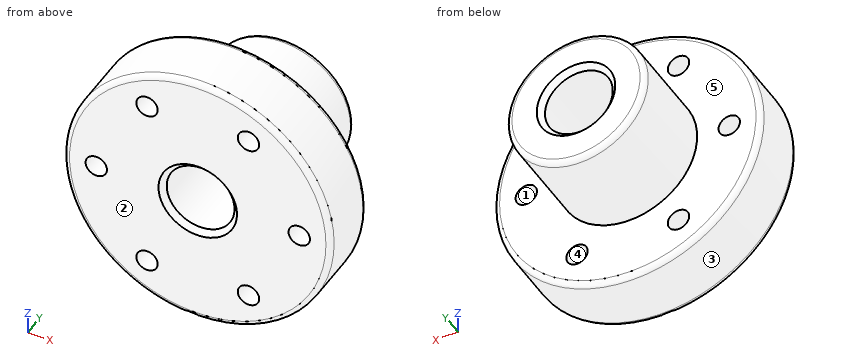
```python
from build123d import *

# Parameters (mm, degrees)
ESQUISSE3_R                  = 1
ENL_V_MAT_EXTRU_1_DEPTH      = 7
R_P_TITION_CIRCULAIRE1_COUNT = 6
CONG_1_R                     = 0.5
CHANFREIN1_SIZE              = 0.5


with BuildPart() as part:
    # Esquisse1 → Révolution2 (revolve)
    with BuildSketch(Plane.XY):
        Polygon((6.5, 15), (6.5, 6), (12.5, 6), (12.5, 0), (3.175, 0), (3.175, 15), align=None)
    revolve(axis=Axis((0, 0, 0), (0, 1, 0)))

    # Esquisse3 → Enlèv. mat.-Extru.1 (cut, through all)
    with BuildSketch(Plane(origin=(0, 6, 0), x_dir=(1, 0, 0), z_dir=(0, 1, 0))):
        with Locations((9.5, 0)):
            Circle(ESQUISSE3_R)
    enl_v_mat_extru_1 = extrude(amount=-ENL_V_MAT_EXTRU_1_DEPTH, mode=Mode.SUBTRACT)

    # Répétition circulaire1: Enlèv. mat.-Extru.1 ×6 about axis
    r_p_tition_circulaire1_axis = Axis((0, 0, 0), (0, 1, 0))
    for i in range(1, R_P_TITION_CIRCULAIRE1_COUNT):
        add(enl_v_mat_extru_1.rotate(r_p_tition_circulaire1_axis, i * 360 / R_P_TITION_CIRCULAIRE1_COUNT), mode=Mode.SUBTRACT)

    # Congé1
    cong_1_edges = [part.edges().sort_by_distance(p)[0] for p in [
        (-6.5, 15, 0),
        (-12.5, 6, 0),
        (-12.5, 0, 0),
    ]]
    fillet(cong_1_edges, radius=CONG_1_R)

    # Chanfrein1
    chanfrein1_edges = [part.edges().sort_by_distance(p)[0] for p in [
        (-3.175, 0, 0),
        (-3.175, 15, 0),
    ]]
    chamfer(chanfrein1_edges, length=CHANFREIN1_SIZE)


solid = part.part
```
Can you work these out from the model? Positions are in its coordinate system, mm. Face numbers are marked on the shaded views. A direction names the side the tool comes from. Coordinates: 2 decimals unless noted, no trailing zeros. Loops run counter-clockwise (first coordinate to the right, second up) from the corner with the lowest first, then second, coordinate; pieces in that order, holes last. Notation, with made-up numbers: (59.5, -26.5) - (102.5, -26.5) arc R35 ccw to (102.5, 6.5) - close; hole circle Ø8 at (-22, 44.25). An arc over 180 degrees is marked (long way). Answer as CSV lines item,"result". Start each with the question number.
1) I need wall thicknesses on line 1 (X direction, y = 9.5, z = 0) (3 decimals); line 2 (X direction, y = 5.25, z = 7.5). Which ranges of each line are inside material? Lowest first, please. Write a range as from..to.
2) Suppose I cut it at C-C (y = 10.75). Please give me the cut outline in (x, z) (3 decimals).
3) For pin 1 (5 mm diameter, centred on x = 8, y = 7.5, fed in from +Z); pin 2 (8 mm diameter, centred on y = 3.5, z = 9, fed in from -X); pin 3 (5.5 mm diameter, centred on x = 0, z = 0, fed in from -Y); pin 4 (2.5 mm diameter, centred on x = 9.5, z = 0, fed in from +Y), each with a flat end and sliding along its axis, tell me the tip position at first contact or that it passes through.
4) Suppose I cut it at A-A (x = 0). Please give me the cut outline in (y, z) (3 decimals), plus the area to 3 significant figures.
5) Which directions (+Z, -Z, +X, -X, +Y, -Y) give clear straight access to the entire face, cutting with the end or side of a thin tool? Please do the marked faces 4 and 5.
6) Suppose I cut it at D-D (x = 4.75). Count the separate pieces of the cut face and the enclosed holes in it, plus the area to 3 significant figures.
7) Suppose I cut it at B-B (y = 1.5). Please give me the cut outline in (x, z) (3 decimals).
8) Thinking about a two-plate mould opening in X: for the marked faces 1, 2 and 3, which applies, pulls with the +X half, pulls with the -X half, needs draft (parallel to the pull), parting line crosses it, or undercut?
Check result:
1,line 1,"x = -6.5..-3.175, 3.175..6.5"
1,line 2,"x = -10..-5.44, -4.06..4.06, 5.44..10"
2,outline,"circle Ø13 at (0, 0); hole circle Ø6.35 at (0, 0)"
3,pin 1,"stops at z = 10.77"
3,pin 2,"stops at x = -11.46"
3,pin 3,"passes through"
3,pin 4,"stops at y = 6"
4,outline,"(0, -12) arc R0.5 ccw to (0.5, -12.5) - (5.5, -12.5) arc R0.5 ccw to (6, -12) - (6, -6.5) - (14.5, -6.5) arc R0.5 ccw to (15, -6) - (15, -3.675) - (14.5, -3.175) - (0.5, -3.175) - (0, -3.675) - close; (0, 3.675) - (0.5, 3.175) - (14.5, 3.175) - (15, 3.675) - (15, 6) arc R0.5 ccw to (14.5, 6.5) - (6, 6.5) - (6, 12) arc R0.5 ccw to (5.5, 12.5) - (0.5, 12.5) arc R0.5 ccw to (0, 12) - close"
4,area,"171 mm²"
5,face 4,"+Y, -Y"
5,face 5,"+Y"
6,separate pieces,"3"
6,enclosed holes,"0"
6,area,"194 mm²"
7,outline,"circle Ø25 at (0, 0); hole circle Ø2 at (-9.5, 0); hole circle Ø2 at (-4.75, -8.227); hole circle Ø2 at (-4.75, 8.227); hole circle Ø6.35 at (0, 0); hole circle Ø2 at (4.75, -8.227); hole circle Ø2 at (4.75, 8.227); hole circle Ø2 at (9.5, 0)"
8,face 1,"undercut"
8,face 2,"needs draft"
8,face 3,"parting line crosses it"
